Work out the finished part from the listing and answer in its coordinate system (mm). Face numbers are marked on the shaded views. A direction names the side the tool comes from. Round coordinates to 2 decimals unless told otherwise and drop trailing zeros. Write each loop counter-clockwise with the first axis right and the second up, starting at its lowest first coordinate (ties: lowest second). Pieces come first, ordered by that corner, then holes. Notation, with made-up numbers: (77, 83.5) -> (83, 83.5) arc R11 cw to (83, 91.5) -> close; hole circle Ø4 at (-18.5, 58.5). An arc over 180 degrees is marked (long way). Answer as a JSON object with one key per item and string values. Group by question number.
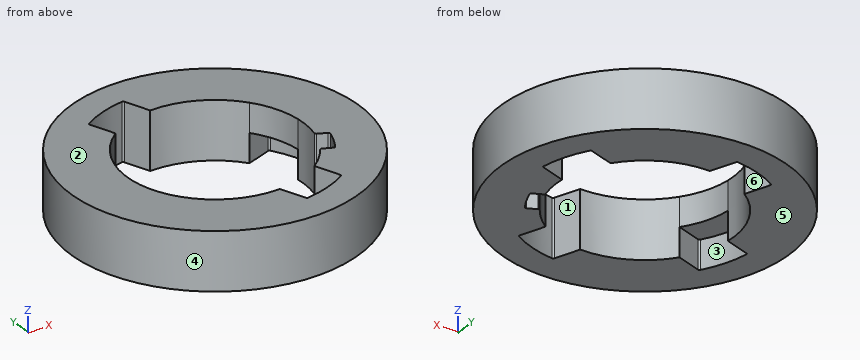
from build123d import *

# Parameters (mm, degrees)
ESQUISSE1_R             = 25
BOSS_EXTRU_1_DEPTH      = 10
ENL_V_MAT_EXTRU_1_DEPTH = 5


with BuildPart() as part:
    # Esquisse1 → Boss.-Extru.1 (new body)
    # profile 1 of 3: a face of its own
    with BuildSketch(Plane.XY):
        Circle(ESQUISSE1_R)
        with BuildLine():
            ThreePointArc((14.787409001, -3.927153556), (14.806182583, -4.132467854), (14.953030626, -4.277181575))
            Line((14.953030626, -4.277181575), (16.501758042, -4.982426557))
            ThreePointArc((16.501758042, -4.982426557), (16.651785463, -5.134087079), (16.663083329, -5.347116418))
            ThreePointArc((16.663083329, -5.347116418), (15.924531384, -7.256672806), (14.968008895, -9.066901881))
            ThreePointArc((14.968008895, -9.066901881), (14.799864591, -9.198133844), (14.587009397, -9.184458985))
            Line((14.587009397, -9.184458985), (13.038282108, -8.478683252))
            ThreePointArc((13.038282108, -8.478683252), (12.832759155, -8.462847948), (12.665533258, -8.583371557))
            ThreePointArc((12.665533258, -8.583371557), (11.047050831, -10.585493278), (9.115784449, -12.28789949))
            Line((9.115784449, -12.28789949), (10.702270918, -16.615013469))
            ThreePointArc((10.702270918, -16.615013469), (10.704320991, -16.815778994), (10.57929488, -16.972876004))
            ThreePointArc((10.57929488, -16.972876004), (6.884626339, -18.777697414), (2.898945402, -19.788787622))
            ThreePointArc((2.898945402, -19.788787622), (2.70200379, -19.749736367), (2.57379576, -19.595225203))
            Line((2.57379576, -19.595225203), (0.987309291, -15.268111225))
            ThreePointArc((0.987309291, -15.268111225), (-6.433398472, -13.881692407), (-12.28789949, -9.115784449))
            Line((-12.28789949, -9.115784449), (-16.615013469, -10.702270918))
            ThreePointArc((-16.615013469, -10.702270918), (-16.815778994, -10.704320991), (-16.972876004, -10.57929488))
            ThreePointArc((-16.972876004, -10.57929488), (-18.777697414, -6.884626339), (-19.788787622, -2.898945402))
            ThreePointArc((-19.788787622, -2.898945402), (-19.749736367, -2.70200379), (-19.595225203, -2.57379576))
            Line((-19.595225203, -2.57379576), (-15.268111225, -0.987309291))
            ThreePointArc((-15.268111225, -0.987309291), (-13.881692407, 6.433398472), (-9.115784449, 12.28789949))
            Line((-9.115784449, 12.28789949), (-10.702270918, 16.615013469))
            ThreePointArc((-10.702270918, 16.615013469), (-10.704320991, 16.815778994), (-10.57929488, 16.972876004))
            ThreePointArc((-10.57929488, 16.972876004), (-6.884626339, 18.777697414), (-2.898945402, 19.788787622))
            ThreePointArc((-2.898945402, 19.788787622), (-2.70200379, 19.749736367), (-2.57379576, 19.595225203))
            Line((-2.57379576, 19.595225203), (-0.987309291, 15.268111225))
            ThreePointArc((-0.987309291, 15.268111225), (6.433398472, 13.881692407), (12.28789949, 9.115784449))
            Line((12.28789949, 9.115784449), (16.615013469, 10.702270918))
            ThreePointArc((16.615013469, 10.702270918), (16.815778994, 10.704320991), (16.972876004, 10.57929488))
            ThreePointArc((16.972876004, 10.57929488), (18.777697414, 6.884626339), (19.788787622, 2.898945402))
            ThreePointArc((19.788787622, 2.898945402), (19.749736367, 2.70200379), (19.595225203, 2.57379576))
            Line((19.595225203, 2.57379576), (15.268111225, 0.987309291))
            ThreePointArc((15.268111225, 0.987309291), (15.227329387, -1.489442759), (14.787409001, -3.927153556))
        make_face(mode=Mode.SUBTRACT)
    # profile 2 of 3: a face of its own
    with BuildSketch(Plane.XY):
        with BuildLine():
            ThreePointArc((12.28789949, 9.115784449), (14.364938522, 5.26673915), (15.268111225, 0.987309291))
            Line((15.268111225, 0.987309291), (19.595225203, 2.57379576))
            ThreePointArc((19.595225203, 2.57379576), (19.749736367, 2.70200379), (19.788787622, 2.898945402))
            ThreePointArc((19.788787622, 2.898945402), (18.777697414, 6.884626339), (16.972876004, 10.57929488))
            ThreePointArc((16.972876004, 10.57929488), (16.815778994, 10.704320991), (16.615013469, 10.702270918))
            Line((16.615013469, 10.702270918), (12.28789949, 9.115784449))
        make_face()
    # profile 3 of 3: a face of its own
    with BuildSketch(Plane.XY):
        with BuildLine():
            ThreePointArc((-12.28789949, -9.115784449), (-14.364938522, -5.26673915), (-15.268111225, -0.987309291))
            Line((-15.268111225, -0.987309291), (-19.595225203, -2.57379576))
            ThreePointArc((-19.595225203, -2.57379576), (-19.749736367, -2.70200379), (-19.788787622, -2.898945402))
            ThreePointArc((-19.788787622, -2.898945402), (-18.777697414, -6.884626339), (-16.972876004, -10.57929488))
            ThreePointArc((-16.972876004, -10.57929488), (-16.815778994, -10.704320991), (-16.615013469, -10.702270918))
            Line((-16.615013469, -10.702270918), (-12.28789949, -9.115784449))
        make_face()
    extrude(amount=BOSS_EXTRU_1_DEPTH)

    # Esquisse1_6 → Enl_v. mat.-Extru.1 (cut)
    with BuildSketch(Plane.XY):
        with BuildLine():
            ThreePointArc((12.28789949, 9.115784449), (14.364938522, 5.26673915), (15.268111225, 0.987309291))
            Line((15.268111225, 0.987309291), (19.595225203, 2.57379576))
            ThreePointArc((19.595225203, 2.57379576), (19.749736367, 2.70200379), (19.788787622, 2.898945402))
            ThreePointArc((19.788787622, 2.898945402), (18.777697414, 6.884626339), (16.972876004, 10.57929488))
            ThreePointArc((16.972876004, 10.57929488), (16.815778994, 10.704320991), (16.615013469, 10.702270918))
            Line((16.615013469, 10.702270918), (12.28789949, 9.115784449))
        make_face()
        with BuildLine():
            ThreePointArc((-12.28789949, -9.115784449), (-14.364938522, -5.26673915), (-15.268111225, -0.987309291))
            Line((-15.268111225, -0.987309291), (-19.595225203, -2.57379576))
            ThreePointArc((-19.595225203, -2.57379576), (-19.749736367, -2.70200379), (-19.788787622, -2.898945402))
            ThreePointArc((-19.788787622, -2.898945402), (-18.777697414, -6.884626339), (-16.972876004, -10.57929488))
            ThreePointArc((-16.972876004, -10.57929488), (-16.815778994, -10.704320991), (-16.615013469, -10.702270918))
            Line((-16.615013469, -10.702270918), (-12.28789949, -9.115784449))
        make_face()
    extrude(amount=ENL_V_MAT_EXTRU_1_DEPTH, mode=Mode.SUBTRACT)


solid = part.part
1) For a pull along Y with two mould halves and no side action, classify the marked faces 4, 5 and 6 as released by +Y, released by -Y, zero draft, split by the parting line, or undercut.
2) Each of these flat-tipped pins is pushed along its axis until it touches: P1, Ø2.5, axis at x = 16.5, y = 6.5, coming from the -Z side; P2, Ø1.5, axis at y = -16.5, z = 4, coming from the +X side; P3, Ø5, axis at x = 7.5, z = 5, coming from the +Y side. Where does it stop, or does it pass through?
3) A cutting plane is placed at B-B on z = 8.25. Determine the outline of the cut face in (x, y).
4) Straight lines are drawn through the part: L1, parallel to X at y = 12, z = 6.25; L2, parallel to Z at x = -15, y = -7.5; L3, parallel to X at y = -12.5, z = 5.5. For each, find the intervals that lie inside material, in ascending order.
5) A cutting plane is placed at A-A on x = 0. Determine the outline of the cut face in (y, z), plus the area to 3 significant figures.
6) A tool of negligible diameter and unlimited length cuts with its end or side. For the marked faces 1, 2 and 3, from which of +Z, -Z, +X, -X, +Y, -Y can it reach the whole face along a straight path? Write none if from no direction.
Established:
{
 "1": {"face 4": "split by the parting line", "face 5": "zero draft", "face 6": "undercut"},
 "2": {"P1": "stops at z = 5", "P2": "stops at x = 19.41", "P3": "stops at y = 24.49"},
 "3": {"outline": "circle Ø50 at (0, 0); hole (-10.7, 16.62) -> (-9.12, 12.29) arc R15.3 ccw to (0.99, -15.27) -> (2.57, -19.6) arc R0.3 ccw to (2.9, -19.79) arc R20 ccw to (10.58, -16.97) arc R0.3 ccw to (10.7, -16.62) -> (9.12, -12.29) arc R15.3 ccw to (12.67, -8.58) arc R0.3 cw to (13.04, -8.48) -> (14.59, -9.18) arc R0.3 ccw to (14.97, -9.07) arc R17.5 ccw to (16.66, -5.35) arc R0.3 ccw to (16.5, -4.98) -> (14.95, -4.28) arc R0.3 cw to (14.79, -3.93) arc R15.3 ccw to (-0.99, 15.27) -> (-2.57, 19.6) arc R0.3 ccw to (-2.9, 19.79) arc R20 ccw to (-10.58, 16.97) arc R0.3 ccw to start"},
 "4": {"L1": "x = -21.93 to -9.49, 9.49 to 21.93", "L2": "z = 5 to 10", "L3": "x = -21.65 to -8.82, 9.19 to 21.65"},
 "5": {"outline": "(-25, 0) -> (-15.3, 0) -> (-15.3, 10) -> (-25, 10) -> close; (15.3, 0) -> (25, 0) -> (25, 10) -> (15.3, 10) -> close", "area": "194 mm²"},
 "6": {"face 1": "+Z, -Z", "face 2": "+Z, +X, -X, +Y, -Y", "face 3": "-Z"}
}
